from build123d import *

# Parameters (mm, degrees)
F1_W     = 23.2
F1_H     = 60
F2_DEPTH = 5
F5_DEPTH = 2
F7_R     = 0.5


with BuildPart() as f2:
    # F1 (on Front) → F2 (new body)
    with BuildSketch(Plane.XZ):
        with Locations((0, -14)):
            Rectangle(F1_W, F1_H)
    extrude(amount=-F2_DEPTH)

    # F4 (on face) → F5 (cut)
    with BuildSketch(Plane.XZ):
        with BuildLine():
            Line((4.5032451175, -39.9769037598), (4.5032451175, 12.0230962402))
            Line((4.5032451175, 12.0230962402), (4.5032451175, 16))
            Line((4.5032451175, 16), (3.5, 16))
            Line((3.5, 16), (3.5, 14.7152424996))
            ThreePointArc((3.5, 14.7152424996), (3.0356981489, 15.2086247741), (2.5025880537, 15.6267107751))
            ThreePointArc((2.5025880537, 15.6267107751), (2.5006470354, 15.5158509267), (2.5, 15.4049759751))
            Line((2.5, 15.4049759751), (2.5, -40))
            ThreePointArc((2.5, -40), (2.8023140413, -41.4229562572), (3.6570311485, -42.6000955676))
            ThreePointArc((3.6570311485, -42.6000955676), (4.2859243089, -41.3548841104), (4.5032451175, -39.9769037598))
        make_face()
    extrude(amount=-F5_DEPTH, mode=Mode.SUBTRACT)

    # F8: sweep along a path in F0
    with BuildLine(Plane.XZ) as f8_path:
        Line((2, 34), (2, 40))
        ThreePointArc((2, 40), (6, 44), (10, 40))
        Line((10, 40), (10, -40))
    # F7 (on plane+point) → F8 (sweep)
    with BuildSketch(Plane.XY.offset(34)):
        with Locations((2, 0)):
            Circle(F7_R)
    sweep(path=f8_path.line)


solid = f2.part
The listing builds one solid part. Answer for the finished solid, in the listing's coordinates (mm). A direction names the side the tool comes from. Coordinates: 2 decimals unless noted, no trailing zeros. Order: outer loops, then holes, each group sorted by start corner. A loop starts at its lowest first (then second) coordinate and runs counter-clockwise, first axis right, second up. Notation, with made-up numbers: (46.5, 11) -> (79.5, 11) arc R17 cw to (79.5, 33) -> close; hole circle Ø11 at (-19.75, -28). An arc over 180 degrees is marked (long way). Answer in a Markdown table with one row per item. Add a question column.
Item 1: Find section C-C (z = 18.5). Write down the section's boundary in (x, y).
Item 2: Determine the mould class of faces 3 (the face through (-11.6, 2, -14)), 4 (the face through (2.5, 1, -12)), 5 (the face through (0, 2, -44)) for opening direction X: +X half, -X half, draft (parallel to the pull), parting line (faces both ways), or undercut.
Item 3: Find the intervals of material crossed by L1, parallel to X at y = 1.3, z = -16.5; L2, parallel to Y at x = 2.25, z = -16; L3, parallel to Z at x = 1.5, y = 0.8, in increasing order. Write a range as from..to.
Item 4: Find section B-B (y = 3.3). Write down the section's boundary in (x, z), then the cut area to 3 significant figures.
Item 5: Which of the six approach directions +Z, -Z, +X, -X, +Y, -Y give full straight-line access (tool end or side, diameter ignored) to faces 1 (the face through (11.6, 2, -14)), 2 (the face through (4.503, 1, -12))?
Item 6: This flat-tipped pin is pushed along its axis until it touches: P1, Ø6, axis at x = -2.5, z = 34, coming from the -Y side. Where does it stop, or does it pass through?
Item 7: Find section A-A (z = -6.5). Write down the section's boundary in (x, y).
Result set:
| question | item | result |
|---|---|---|
| 1 | outline | circle Ø1 at (10, 0) |
| 2 | face 3 | -X half |
| 2 | face 4 | undercut |
| 2 | face 5 | draft |
| 3 | L1 | x = -11.6..2.5, 4.5..11.6 |
| 3 | L2 | y = 0..5 |
| 3 | L3 | z = -44..16 |
| 4 | outline | (-11.6, -44) -> (11.6, -44) -> (11.6, 16) -> (-11.6, 16) -> close |
| 4 | area | 1,390 mm² |
| 5 | face 1 | +Z, -Z, +X, +Y, -Y |
| 5 | face 2 | -Y |
| 6 | P1 | passes through |
| 7 | outline | (-11.6, 0) -> (2.5, 0) -> (2.5, 2) -> (4.5, 2) -> (4.5, 0) -> (9.5, 0) arc R0.5 ccw to (10.5, 0) -> (11.6, 0) -> (11.6, 5) -> (-11.6, 5) -> close |
